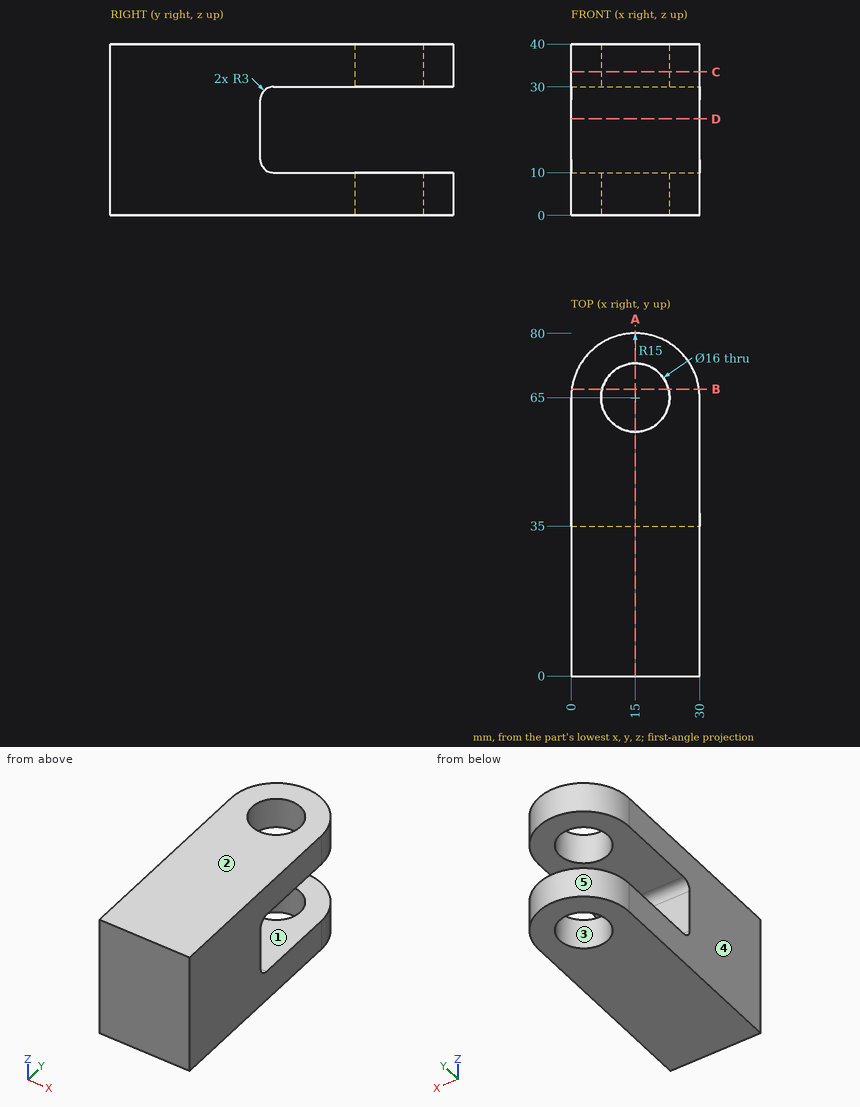
Geometry check sheet. Reference: drawing and pictorial views, mm from the part's lowest x, y, z. A direction names the side the tool comes from. Give positions to 0.01 mm unless a question says otherwise; leave off trailing zeros. Loops run counter-clockwise (first coordinate to the right, second up) from the corner with the lowest first, then second, coordinate; pieces in that order, holes last.
1. Section check C-C, the plane z = 33.5. Enter the section's corners in (x, y), then the cut area to 3 significant figures.
2. Section check A-A, the plane x = 15. Enter the section's corners in (y, z).
3. Section check D-D, the plane z = 22.5. Enter the section's corners in (x, y).
4. Mould release check, pull along Y, two halves, no side actions. Record for the marked faces 3, 4 and 5: released by +Y, released by -Y, zero draft, split by the parting line, or undercut.
5. Go/stop test with flat-tipped pins: pin 1 Ø7 at (x, z) = (11.5, 16.5) entering from +Y; pin 2 Ø9.5 at (x, y) = (15, 65) entering from -Z; pin 3 Ø1.5 at (x, z) = (24, 4) entering from +Y. Record where each tip stops, or that it passes through.
6. Thickness scan on line 1 (X direction, y = 65, z = 35); line 2 (Y direction, x = 15, z = 35); line 3 (Z direction, x = 22.5, y = 53). Record the ranges inside material, lowest first.
7. Set-up check for the marked faces 1 and 2: record each of +Z, -Z, +X, -X, +Y, -Y from which the full face is reachable in a straight line by a thin tool's end or side.
8. Section check B-B, the plane y = 67. Enter the section's corners in (x, z), then the cut area to 3 significant figures.
Geometry says:
1. outline: (0, 0) - (30, 0) - (30, 65) arc R15 ccw to (0, 65) - close; hole circle Ø16 at (15, 65)
1. area: 2,100 mm2
2. outline: (0, 0) - (57, 0) - (57, 10) - (38, 10) arc R3 cw to (35, 13) - (35, 27) arc R3 cw to (38, 30) - (57, 30) - (57, 40) - (0, 40) - close; (73, 0) - (80, 0) - (80, 10) - (73, 10) - close; (73, 30) - (80, 30) - (80, 40) - (73, 40) - close
3. outline: (0, 0) - (30, 0) - (30, 35) - (0, 35) - close
4. face 3: undercut
4. face 4: zero draft
4. face 5: released by +Y
5. pin 1: stops at y = 35
5. pin 2: passes through
5. pin 3: stops at y = 77.53
6. line 1: x = 0 to 7, 23 to 30
6. line 2: y = 0 to 57, 73 to 80
6. line 3: z = 0 to 10, 30 to 40
7. face 1: +X, -X, +Y
7. face 2: +Z, +X, -X, +Y, -Y
8. outline: (0.13, 0) - (7.25, 0) - (7.25, 10) - (0.13, 10) - close; (0.13, 30) - (7.25, 30) - (7.25, 40) - (0.13, 40) - close; (22.75, 0) - (29.87, 0) - (29.87, 10) - (22.75, 10) - close; (22.75, 30) - (29.87, 30) - (29.87, 40) - (22.75, 40) - close
8. area: 285 mm2
